Check sheet for the modelled part. Datum: model origin and axes. Units: mm. A direction names the side the tool comes from. Round coordinates to 2 decimals unless told otherwise and drop trailing zeros. Loops run counter-clockwise (first coordinate to the right, second up) from the corner with the lowest first, then second, coordinate; pieces in that order, holes last. Notation, with made-up numbers: M 53,-24 L 108,-24 A31 cw 108,4 Z; hole C 86,-5 d5. An arc over 180 degrees is marked long. One line per question, with ' | ' between items. Start each with the question number.
(1) Draft check along X on faces 4 (the face through (0.444, -6, 2)), 5 (the face through (-4, -25.556, 2)), 6 (the face through (77.694, -11, 2)), 7 (the face through (-52.806, -18, 2)). Enter one of: +X half, -X half, draft (parallel to the pull), parting line (faces both ways), or undercut.
(2) Tool access check on faces 1 (the face through (76, 14.444, 2)), 2 (the face through (-28, -13.556, 2)), 3 (the face through (13, 18, 0)). Record the directions out of +Z, -Z, +X, -X, +Y, -Y that give a thin tool (end or side, any length) a straight path to the whole face; none if there is none.
(3) Section check B-B (y = -18). Record the boundary of the cut face in (x, z), and give its area (4 significant figures).
(4) Section check C-C (x = 14.5). Record the boundary of the cut face in (y, z).
(5) Go/stop test with flat-tipped pins: P1, Ø1.5, axis at y = -16.5, z = 1.5, coming from the +X side; P2, Ø1, axis at y = -10, z = 1, coming from the -X side. Record where each tip stops, or that it passes through.
(6) Section check D-D (z = 2.05). Count the separate pieces of the cut face and the enclosed holes in it, and give its area (3 significant figures).
(7) Section check A-A (y = 18.5). Record the boundary of the cut face in (x, z), and give its area (3 significant figures).
(8) Thickness scan on probe 1 along X at (y, z) = (-23, 0.4); probe 2 along X at (y, z) = (18, 2.9); probe 3 along X at (y, z) = (-7, 1.1). Record the ranges inside material, lowest first. Write a range as [from, to].
```python
from build123d import *

# Parameters (mm, degrees)
F0_W      = 3.5
F0_H      = 10
F1_DEPTH  = 3.5
F1_FACE_W = 60
F1_FACE_H = 3.5
F2_DEPTH  = 3.5
F4_DEPTH  = 3.5
F5_W      = 10
F5_H      = 3.5
F6_DEPTH  = 3.5
F7_W      = 3.5
F7_H      = 10
F8_DEPTH  = 3.5


with BuildPart() as f1:
    # F0 (on Top) → F1 (new body)
    with BuildSketch(Plane.XY):
        Polygon((-49.305556, 34.444444), (-49.305556, -25.555556), (-23.555556, -25.555556), (-23.555556, 14.444444), (-7.555556, 14.444444), (-7.555556, -25.555556), (-5.305556, -25.555556), (-1.805556, -25.555556), (0.444444, -25.555556), (0.444444, 14.444444), (16.444444, 14.444444), (16.444444, -25.555556), (74.194444, -25.555556), (74.194444, 34.444444), (-1.805556, 34.444444), (-5.305556, 34.444444), align=None)
        with Locations((-3.555556, -10.555556)):
            Rectangle(F0_W, F0_H, mode=Mode.SUBTRACT)
        with Locations((-3.555556, 19.444444)):
            Rectangle(F0_W, F0_H, mode=Mode.SUBTRACT)
    extrude(amount=F1_DEPTH)

    # F1_face (on face) → F2 (join)
    with BuildSketch(Plane(origin=(-49.305556, 4.444444, 1.75), x_dir=(0, -1, 0), z_dir=(-1, 0, 0))):
        Rectangle(F1_FACE_W, F1_FACE_H)
    extrude(amount=F2_DEPTH)

    # F3 (on face) → F4 (cut)
    with BuildSketch(Plane.XY.offset(3.5)):
        Polygon((-49.305556, 22.444444), (-52.805556, 20.444444), (-52.805556, 14.444444), (-49.305556, 12.444444), align=None)
        Polygon((-49.305556, -3.555556), (-52.805556, -5.555556), (-52.805556, -11.555556), (-49.305556, -13.555556), align=None)
    extrude(amount=-F4_DEPTH, mode=Mode.SUBTRACT)

    # F5 (on face) → F6 (join)
    with BuildSketch(Plane.YZ.offset(74.194444)):
        with Locations((-10.555556, 1.75)):
            Rectangle(F5_W, F5_H)
        with Locations((19.444444, 1.75)):
            Rectangle(F5_W, F5_H)
    extrude(amount=F6_DEPTH)

    # F7 (on face) → F8 (cut)
    with BuildSketch(Plane.XY.offset(3.5)):
        with Locations((-27.555556, 17.444444)):
            Rectangle(F7_W, F7_H)
        with Locations((-27.555556, -8.555556)):
            Rectangle(F7_W, F7_H)
    extrude(amount=-F8_DEPTH, mode=Mode.SUBTRACT)


solid = f1.part
```
The answers:
1) face 4: undercut | face 5: draft | face 6: +X half | face 7: -X half
2) face 1: +Z, -Z, +X | face 2: +Z, -Z | face 3: -Z, +X, -X, +Y, -Y
3) outline: M -52.81,0 L -23.56,0 L -23.56,3.5 L -52.81,3.5 Z; M -7.56,0 L 0.44,0 L 0.44,3.5 L -7.56,3.5 Z; M 16.44,0 L 74.19,0 L 74.19,3.5 L 16.44,3.5 Z | area: 332.5 mm²
4) outline: M 14.44,0 L 34.44,0 L 34.44,3.5 L 14.44,3.5 Z
5) P1: x = 74.19 | P2: x = -49.31
6) separate pieces: 1 | enclosed holes: 4 | area: 6,210 mm²
7) outline: M -49.31,0 L -29.31,0 L -29.31,3.5 L -49.31,3.5 Z; M -25.81,0 L -5.31,0 L -5.31,3.5 L -25.81,3.5 Z; M -1.81,0 L 77.69,0 L 77.69,3.5 L -1.81,3.5 Z | area: 420 mm²
8) probe 1: [-52.81, -23.56], [-7.56, 0.44], [16.44, 74.19] | probe 2: [-49.31, -29.31], [-25.81, -5.31], [-1.81, 77.69] | probe 3: [-49.31, -29.31], [-25.81, -23.56], [-7.56, -5.31], [-1.81, 0.44], [16.44, 77.69]
